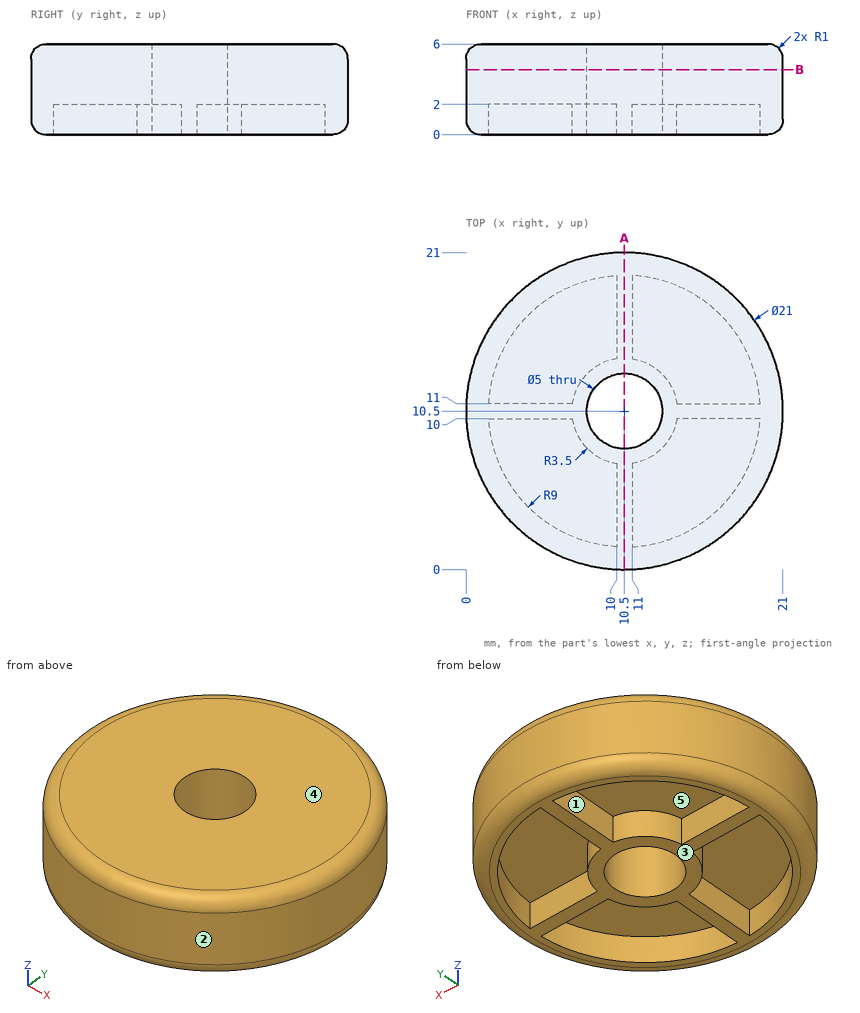
Source: three-view drawing plus pictorial views. Frame: mm from the lowest corner of the part. A direction names the side the tool comes from. Give positions to 0.01 mm unless a question says otherwise; leave off trailing zeros. Order: outer loops, then holes, each group sorted by start corner. A loop starts at its lowest first (then second) coordinate and runs counter-clockwise, first axis right, second up. Notation, with made-up numbers: M 2.5,2.5 L 28.5,2.5 A30 ccw 28.5,29.5 Z; hole C 68,-21.75 d5. An arc over 180 degrees is marked long. One line per question, with ' | ' between items.
1) Section A-A on x = 10.5. Output: boundary loops of the cut face in (y, z).
Filled in:
outline: M 0,1 A1 ccw 1,0 L 8,0 L 8,6 L 1,6 A1 ccw 0,5 Z; M 13,0 L 20,0 A1 ccw 21,1 L 21,5 A1 ccw 20,6 L 13,6 Z
2) Contact query for flat-ended pins moving along their axis: P1, Ø1, axis at x = 16, z = 1, coming from the -Y side; P2, Ø1, axis at y = 4.5, z = 1.5, coming from the -X side; P3, Ø0.6, axis at x = 4, z = 1, coming from the +Y side. Output: stop coordinate, or through.
Filled in:
P1: stops at y = 1.27 | P2: stops at x = 1.56 | P3: stops at y = 18.97
3) Access query for the marked faces 4 and 5. Directions: +Z, -Z, +X, -X, +Y, -Y. A direction counts if a zero-diameter tool reaches every point of the face in a straight line with its end or side. Return the directions, or none.
Filled in:
face 4: +Z, +X, -X, +Y, -Y | face 5: -Z
4) Ray query, L1, parallel to Y at x = 6.5, z = 1; L2, parallel to Y at x = 10.5, z = 3.6; L3, parallel to Y at x = 5, z = 1.5. Return the intervals inside material, ascending.
Filled in:
L1: y = 0.79 to 2.44, 10 to 11, 18.56 to 20.21 | L2: y = 0 to 8, 13 to 21 | L3: y = 1.56 to 3.38, 10 to 11, 17.62 to 19.44
5) Section B-B on z = 4.3. Output: boundary loops of the cut face in (x, y).
Filled in:
outline: C 10.5,10.5 d21; hole C 10.5,10.5 d5
6) Draft query along X for the marked faces 1, 2 and 3. Return one class per face: pulls with the +X half, pulls with the -X half, needs draft (parallel to the pull), parting line crosses it, or undercut.
Filled in:
face 1: undercut | face 2: parting line crosses it | face 3: needs draft
